The model under review builds one solid part; all positions refer to its coordinate system, in mm. Coordinates: 2 decimals unless noted, no trailing zeros. Loops run counter-clockwise (first coordinate to the right, second up) from the corner with the lowest first, then second, coordinate; pieces in that order, holes last. Notation, with made-up numbers: M 72.5,-3.5 L 94.5,-3.5 A24 cw 94.5,29.5 Z; hole C 9,-28 d1. An arc over 180 degrees is marked long. Write item = value, one per line. Start each with the question number.
Q1. Wall thickness on probe 1 along Y at (x, z) = (122, 1.65); probe 2 along Y at (x, z) = (133.5, 2.65); probe 3 along X at (y, z) = (212, 1.7): over which ranges is each line inside the solid? List them lowest first.
Q2. We need section C-C on z = 1.5. Count the separate pieces of the cut face and the enclosed holes in it, and give its area (3 significant figures).
Q3. Clearance check with a flat-ended pin moving along its axis: pin 1 Ø2.5 at (x, y) = (109.12, 223.9) entering from +Z. State where the tip first meets the part, or that it passes through.
Q4. We need section B-B on x = 134. Give the boundary of the cut face in (y, z).
Q5. We need section D-D on x = 114. Give the boundary of the cut face in (y, z).
Q6. We need section A-A on y = 216.75. Give the boundary of the cut face in (x, z), and give its area (3 significant figures).
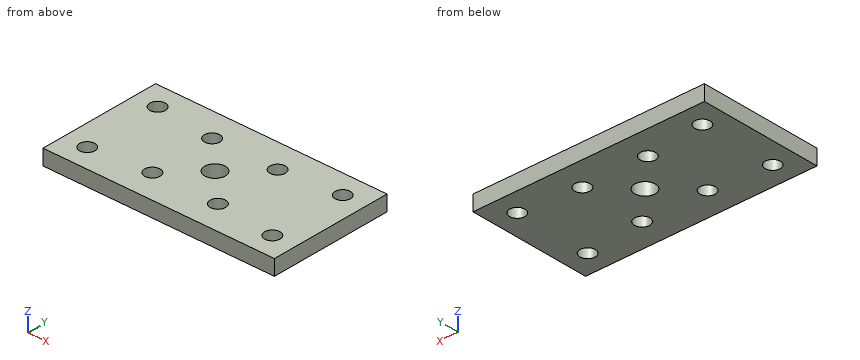
from build123d import *

# Parameters (mm, degrees)
MODEL_R                 = 1.5
MODEL_R_2               = 2
SALIENTE_EXTRUIR1_DEPTH = 3


with BuildPart() as part:
    # Model → Saliente-Extruir1 (new body)
    with BuildSketch(Plane.XY):
        Polygon((92.985593985, 229.537066641), (137.985593985, 229.537057995), (137.985593985, 205.537057995), (92.985593985, 205.537066641), align=None)
        with Locations((109.121632955, 223.901023349)):
            Circle(MODEL_R, mode=Mode.SUBTRACT)
        with Locations((121.849555016, 211.173101287)):
            Circle(MODEL_R, mode=Mode.SUBTRACT)
        with Locations((121.849555016, 223.901023349)):
            Circle(MODEL_R, mode=Mode.SUBTRACT)
        with Locations((109.121632955, 211.173101287)):
            Circle(MODEL_R, mode=Mode.SUBTRACT)
        with Locations((115.485593985, 217.537062318)):
            Circle(MODEL_R_2, mode=Mode.SUBTRACT)
        with Locations((97.485593985, 225.037066641)):
            Circle(MODEL_R, mode=Mode.SUBTRACT)
        with Locations((97.485593985, 210.037066641)):
            Circle(MODEL_R, mode=Mode.SUBTRACT)
        with Locations((133.485593985, 225.037057995)):
            Circle(MODEL_R, mode=Mode.SUBTRACT)
        with Locations((133.485593985, 210.037057995)):
            Circle(MODEL_R, mode=Mode.SUBTRACT)
    extrude(amount=SALIENTE_EXTRUIR1_DEPTH)


solid = part.part
Returned:
q1.probe_1 = 205.54 to 209.68, 212.67 to 222.41, 225.39 to 229.54
q1.probe_2 = 205.54 to 208.54, 211.54 to 223.54, 226.54 to 229.54
q1.probe_3 = 92.99 to 107.87, 110.37 to 120.6, 123.1 to 137.99
q2.separate_pieces = 1
q2.enclosed_holes = 9
q2.area = 1,010 mm^2
q3.pin_1 = through
q4.outline = M 205.54,0 L 208.63,0 L 208.63,3 L 205.54,3 Z; M 211.45,0 L 223.63,0 L 223.63,3 L 211.45,3 Z; M 226.45,0 L 229.54,0 L 229.54,3 L 226.45,3 Z
q5.outline = M 205.54,0 L 216.2,0 L 216.2,3 L 205.54,3 Z; M 218.88,0 L 229.54,0 L 229.54,3 L 218.88,3 Z
q6.outline = M 92.99,0 L 113.65,0 L 113.65,3 L 92.99,3 Z; M 117.32,0 L 137.99,0 L 137.99,3 L 117.32,3 Z
q6.area = 124 mm^2
